Answer from the drawing. Dimensions are ordinates in mm from the lowest x, y and z of the part. A direction names the side the tool comes from. Give positions to 0.01 mm unless a question says otherwise; leave off trailing zeros. Order: outer loops, then holes, each group sorted by start corner. A loop starts at its lowest first (then second) coordinate and runs counter-clockwise, first axis right, second up. Notation, with made-up numbers: M 26,29.25 L 30,29.25 A31 cw 30,59.25 Z; hole C 87.25,17 d3. An arc over 180 degrees is marked long. One line per item, written item: value.
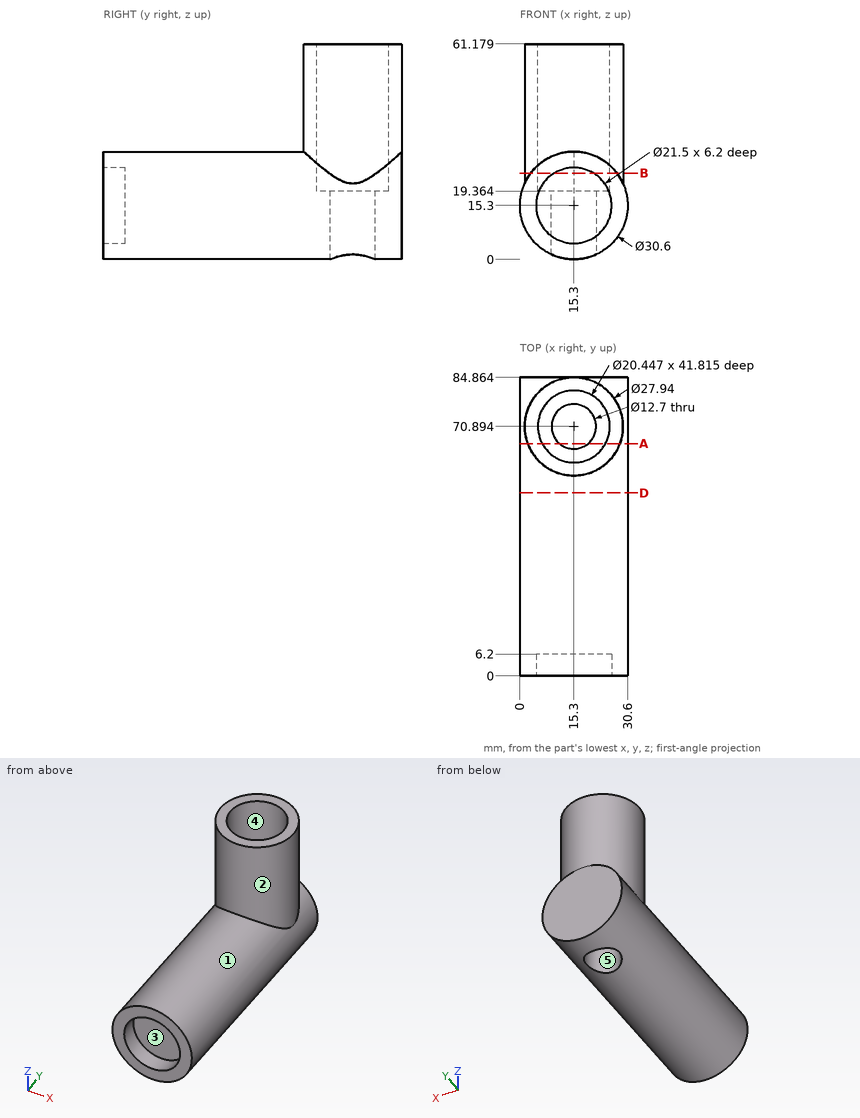
(1) Section B-B, the plane z = 24.5 is taken. Give the vertices of the cut face in (x, y) (1 decimal).
Findings:
outline: M 3.1,0 L 9.7,0 L 9.7,6.2 L 20.9,6.2 L 20.9,0 L 27.5,0 L 27.5,64.1 A14 ccw 27.5,77.7 L 27.5,84.9 L 3.1,84.9 L 3.1,77.7 A14 ccw 3.1,64.1 Z; hole C 15.3,70.9 d20.4
(2) Section D-D, the plane y = 52 is taken. Give the vertices of the cut face in (x, z).
Findings:
outline: C 15.3,15.3 d30.6
(3) Determine the mould class of the marked faces 1, 2 and 3 for opening direction Z: pulls with the +Z half, pulls with the -Z half, needs draft (parallel to the pull), parting line crosses it, or undercut.
Findings:
face 1: parting line crosses it
face 2: needs draft
face 3: undercut
(4) Section A-A, the plane y = 66 is taken. Give the vertices of the cut face in (x, z) (1 decimal), then the cut area to 3 significant figures.
Findings:
outline: M 2.2,23.2 A15.3 ccw 11.3,0.5 L 11.3,19.4 L 6.3,19.4 L 6.3,61.2 L 2.2,61.2 Z; M 19.3,0.5 A15.3 ccw 28.4,23.2 L 28.4,61.2 L 24.3,61.2 L 24.3,19.4 L 19.3,19.4 Z
area: 686 mm^2
(5) Which of the six approach directions +Z, -Z, +X, -X, +Y, -Y give full straight-line access (tool end or side, diameter ignored) to the marked faces 4 and 5?
Findings:
face 4: +Z
face 5: +Z, -Z
(6) Given P1, Ø17, axis at x = 15.3, z = 15.3, coming from the -Y side; P2, Ø3, axis at x = 11.5, z = 42, coming from the -Y side (1 decimal); P3, Ø8, axis at x = 22.5, y = 26.5, coming from the -Z side; P4, Ø2, axis at y = 20.5, z = 15, coming from the -X side, each flat-ended and moving along its own axis, determine where each tip first touches the part or whether it passes through.
Findings:
P1: stops at y = 6.2
P2: stops at y = 57.1
P3: stops at z = 0.34
P4: stops at x = 0
(7) Find the intervals of material crossed by probe 1 along X at (y, z) = (3, 15); probe 2 along Z at (x, y) = (15, 79), in increasing order. Write a range as from..to.
Findings:
probe 1: x = 0..4.55, 26.05..30.6
probe 2: z = 0..19.36
